Here's how the part is built. I have some questions about the finished solid (model axes, mm). Face numbers are marked on the shaded views. A direction names the side the tool comes from. Round coordinates to 2 decimals unless told otherwise and drop trailing zeros. Write each loop counter-clockwise with the first axis right and the second up, starting at its lowest first coordinate (ties: lowest second). Pieces come first, ordered by that corner, then holes. Notation, with made-up numbers: (74, 75.25) -> (133, 75.25) arc R19 cw to (133, 97.25) -> close; hole circle Ø9 at (70.25, -15.5). An arc over 180 degrees is marked (long way). Answer as CSV lines item,"result".
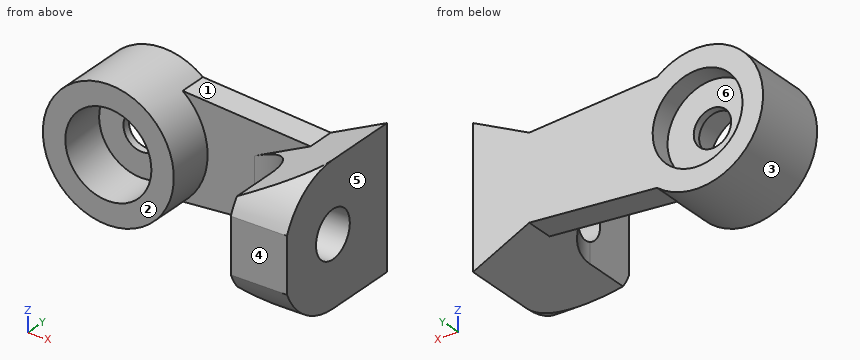
from build123d import *

# Parameters (mm, degrees)
SKETCH_1_R               = 3.5
EXTRUDE_1_DEPTH          = 4
SKETCH_2_R               = 2.4
CUT_EXTRUDE_1_DEPTH      = 1.1
SKETCH_3_R               = 1
CUT_EXTRUDE_2_DEPTH      = 6.736723804
SKETCH_4_R               = 2.3
CUT_EXTRUDE_3_DEPTH      = 2.5
EXTRUDE_START            = -1.5
EXTRUDE_2_DEPTH          = 1.5
EXTRUDE_3_DEPTH          = 7.4
CUT_EXTRUDE_4_DEPTH      = 17.902366698
CUT_EXTRUDE_4_DEPTH_BACK = 17.902366698
SKETCH_10_R              = 1.25
CUT_EXTRUDE_5_DEPTH      = 7.4


with BuildPart() as part:
    # Эскиз1 → Бобышка-Вытянуть1 (new body)
    with BuildSketch(Plane(origin=(0, 0, 0), x_dir=(1, 0, 0), z_dir=(0, 1, 0))):
        with Locations(Location((0, 0, 0), (0, 0, 270))):
            Circle(SKETCH_1_R)
    extrude(amount=EXTRUDE_1_DEPTH)

    # Эскиз2 → Вырез-Вытянуть1 (cut)
    with BuildSketch(Plane(origin=(0, 4, 0), x_dir=(1, 0, 0), z_dir=(0, 1, 0))):
        with Locations(Location((0, 0, 0), (0, 0, 270))):
            Circle(SKETCH_2_R)
    extrude(amount=-CUT_EXTRUDE_1_DEPTH, mode=Mode.SUBTRACT)

    # Эскиз3 → Вырез-Вытянуть2 (cut, through all)
    with BuildSketch(Plane(origin=(0, 2.9, 0), x_dir=(1, 0, 0), z_dir=(0, 1, 0))):
        with Locations(Location((0, 0, 0), (0, 0, 270))):
            Circle(SKETCH_3_R)
    extrude(amount=-CUT_EXTRUDE_2_DEPTH, mode=Mode.SUBTRACT)

    # Эскиз4 → Вырез-Вытянуть3 (cut)
    with BuildSketch(Plane(origin=(0, 0, 0), x_dir=(-1, 0, 0), z_dir=(0, -1, 0))):
        with Locations(Location((0, 0, 0), (0, 0, 90))):
            Circle(SKETCH_4_R)
    extrude(amount=-CUT_EXTRUDE_3_DEPTH, mode=Mode.SUBTRACT)

    # Эскиз5 → Бобышка-Вытянуть2 (add)
    with BuildSketch(Plane(origin=(0, 4, 0), x_dir=(1, 0, 0), z_dir=(0, 1, 0)).offset(EXTRUDE_START)):
        with BuildLine():
            Line((14.15, 1.85), (2.165063509, 2.75))
            ThreePointArc((2.165063509, 2.75), (3.5, 0), (2.165063509, -2.75))
            Line((2.165063509, -2.75), (14.15, -1.85))
            ThreePointArc((14.15, -1.85), (16, 0), (14.15, 1.85))
        make_face()
    extrude(amount=EXTRUDE_2_DEPTH)

    # Эскиз6 → Бобышка-Вытянуть3 (add)
    with BuildSketch(Plane(origin=(0, 4, 0), x_dir=(1, 0, 0), z_dir=(0, 1, 0))):
        Polygon((12, 0), (12, 3.7), (4.4, 0), (12, -3.7), align=None)
    extrude(amount=-EXTRUDE_3_DEPTH)

    # Эскиз9 → Вырез-Вытянуть4 (cut, two sides: drawn at the far end of the back side and taken through both)
    with BuildSketch(Plane.XY.offset(-CUT_EXTRUDE_4_DEPTH_BACK)):
        with BuildLine():
            ThreePointArc((5.997603859, 2.5), (8.11804802, 1.622196165), (8.997602836, -0.497522293))
            Line((8.997602836, -0.497522293), (9, -3.4))
            Line((9, -3.4), (2.724891775, -4.807995463))
            Line((2.724891775, -4.807995463), (4.4, 2.5))
            Line((4.4, 2.5), (5.997603859, 2.5))
        make_face()
        Polygon((17.66550591, -1.447270523), (12, 2.5), (12, 6.114360592), (17.66550591, 6.114360592), align=None)
    extrude(amount=CUT_EXTRUDE_4_DEPTH + CUT_EXTRUDE_4_DEPTH_BACK, mode=Mode.SUBTRACT)

    # Эскиз10 → Вырез-Вытянуть5 (cut)
    with BuildSketch(Plane(origin=(12, 0, 0), x_dir=(0, 0, -1), z_dir=(1, 0, 0))):
        Circle(SKETCH_10_R)
        with BuildLine():
            Line((-3.7, 0), (-6.427289466, -4.290908474))
            Line((-6.427289466, -4.290908474), (7.207363266, -4.845162651))
            Line((7.207363266, -4.845162651), (3.7, 0))
            ThreePointArc((3.7, 0), (0, -3.7), (-3.7, 0))
        make_face()
    extrude(amount=-CUT_EXTRUDE_5_DEPTH, mode=Mode.SUBTRACT)


solid = part.part
Item 1: Will these pins go through, and if not, where does the flat tip stop? pin 1 (3 mm diameter, centred on x = 4, z = 1, fed in from -Y); pin 2 (1.4 mm diameter, centred on x = -0.5, z = 1, fed in from +Y); pin 3 (2.5 mm diameter, centred on x = 0, z = 0, fed in from -Y); pin 4 (3 mm diameter, centred on y = 0, z = 0, fed in from +X).
Results found:
pin 1,"stops at y = 0"
pin 2,"stops at y = 2.9"
pin 3,"stops at y = 2.5"
pin 4,"stops at x = 12"
Item 2: If we mould it in two halves opening along X, with no side actions, what happens to the marked faces 4, 5 and 6? For each: pulls with the +X half, pulls with the -X half, needs draft (parallel to the pull), parting line crosses it, or undercut.
Results found:
face 4,"needs draft"
face 5,"pulls with the +X half"
face 6,"undercut"
Item 3: I need wall thicknesses on L1, parallel to X at y = 0.8, z = 0; L2, parallel to Y at x = 9.3, z = 0; L3, parallel to X at y = 1.4, z = 0. Which ranges of each line are inside material? Lowest first, please.
Results found:
L1,"x = -3.5 to -2.3, 2.3 to 3.5"
L2,"y = -3.4 to -1.25, 1.25 to 4"
L3,"x = -3.5 to -2.3, 2.3 to 3.5, 8.32 to 12"
Item 4: Suppose I cut it at C-C, the plane z = 0.5. List the corners of the cut face in (x, y) for me (3 decimals), then the cut area to 3 significant figures.
Results found:
outline,"(-3.464, 0) -> (-2.245, 0) -> (-2.245, 2.5) -> (-0.866, 2.5) -> (-0.866, 2.9) -> (-2.347, 2.9) -> (-2.347, 4) -> (-3.464, 4) -> close; (0.866, 2.5) -> (2.245, 2.5) -> (2.245, 0) -> (3.464, 0) -> (3.464, 2.5) -> (5.998, 2.5) arc R3 cw to (8.506, 1.146) -> (12, 1.146) -> (12, 4) -> (2.347, 4) -> (2.347, 2.9) -> (0.866, 2.9) -> close; (8.998, -1.146) -> (9, -3.4) -> (12, -3.4) -> (12, -1.146) -> close"
area,"35.9 mm²"
Item 5: For the marked faces 1, 2 and 3, which set-ups out of +Z, -Z, +X, -X, +Y, -Y let a thin tool reach every point of the face, with its end or its side?
Results found:
face 1,"+Z, +Y, -Y"
face 2,"+Z, -Z, -X, -Y"
face 3,"-Y"
Item 6: Suppose I cut it at A-A, the plane y = 3.5. List the corners of the cut face in (x, z) for me, then the cut area to 3 significant figures.
Results found:
outline,"(2.17, -2.75) -> (9, -2.24) -> (12, -3.7) -> (12, 3.7) -> (9, 2.24) -> (2.17, 2.75) arc R3.5 ccw (long way) to start; hole circle Ø4.8 at (0, 0)"
area,"67.2 mm²"
Item 7: Suppose I cut it at B-B, the plane x = 0. List the corners of the cut face in (y, z) for me.
Results found:
outline,"(0, -3.5) -> (4, -3.5) -> (4, -2.4) -> (2.9, -2.4) -> (2.9, -1) -> (2.5, -1) -> (2.5, -2.3) -> (0, -2.3) -> close; (0, 2.3) -> (2.5, 2.3) -> (2.5, 1) -> (2.9, 1) -> (2.9, 2.4) -> (4, 2.4) -> (4, 3.5) -> (0, 3.5) -> close"
Item 8: Suppose I cut it at D-D, the plane z = -3. List the corners of the cut face in (x, y) for me, then the cut area to 3 significant figures.
Results found:
outline,"(-1.8, 0) -> (1.8, 0) -> (1.8, 4) -> (-1.8, 4) -> close; (10.56, -2.17) -> (12, -2.17) -> (12, 4) -> (10.56, 4) -> close"
area,"23.3 mm²"
